Could you check a few things on this model? Use its own coordinates, in mm. Give positions to 0.01 mm unless a question says otherwise; leave off trailing zeros. Loops run counter-clockwise (first coordinate to the right, second up) from the corner with the lowest first, then second, coordinate; pieces in that order, holes last. Notation, with made-up numbers: M 19,5.25 L 58,5.25 A23 ccw 58,37.25 Z; hole C 7,28 d4. An arc over 180 degrees is marked long. Answer in a Markdown table with one row per item. Add a question column.
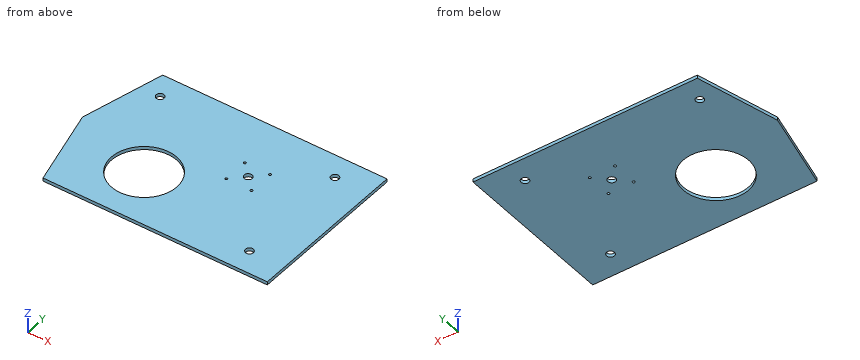
```python
from build123d import *

# Parameters (mm, degrees)
SKETCH1_R           = 40
SKETCH1_R_2         = 4.8
SKETCH1_R_3         = 1.5
BOSS_EXTRUDE3_DEPTH = 4


with BuildPart() as part:
    # Sketch1 → Boss-Extrude3 (new body)
    with BuildSketch(Plane.XY):
        Polygon((-125, -100), (150, -100), (150, 100), (-125, 100), (-150, 0), align=None)
        with Locations((-50, -33.333333333)):
            Circle(SKETCH1_R, mode=Mode.SUBTRACT)
        with Locations((107.142857143, -71.428571429)):
            Circle(SKETCH1_R_2, mode=Mode.SUBTRACT)
        with Locations((-107.142857143, 71.428571429)):
            Circle(SKETCH1_R_2, mode=Mode.SUBTRACT)
        with Locations((21.832408692, 6.152026506)):
            Circle(SKETCH1_R_3, mode=Mode.SUBTRACT)
        with Locations((37.332408692, 21.652026506)):
            Circle(SKETCH1_R_2, mode=Mode.SUBTRACT)
        with Locations((52.832408692, 6.152026506)):
            Circle(SKETCH1_R_3, mode=Mode.SUBTRACT)
        with Locations((21.832408692, 37.152026506)):
            Circle(SKETCH1_R_3, mode=Mode.SUBTRACT)
        with Locations((52.832408692, 37.152026506)):
            Circle(SKETCH1_R_3, mode=Mode.SUBTRACT)
        with Locations((107.142857143, 71.428571429)):
            Circle(SKETCH1_R_2, mode=Mode.SUBTRACT)
    extrude(amount=BOSS_EXTRUDE3_DEPTH)


solid = part.part
```
Item 1: Suppose I cut it at A-A (x = -50). List the corners of the cut face in (y, z) for me.
Item 2: For P1, Ø2.5, axis at x = 21.83, y = 6.15, coming from the +Z side, with a flat end and sliding along its axis, tell me the tip position at first contact or that it passes through.
Item 3: Suppose I cut it at C-C (z = 3.1). Give the number of separate pieces and of enclosed holes in the cut face, then the cut area to 3 significant figures.
Item 4: Suppose I cut it at D-D (y = 87). List the corners of the cut face in (x, z) for me.
Item 5: Suppose I cut it at B-B (y = -29). List the corners of the cut face in (x, z) for me, then the cut area to 3 significant figures.
Item 6: I need wall thicknesses on L1, parallel to X at y = 70, z = 3.65; L2, parallel to X at y = 67, z = 0.5; L3, parallel to Y at x = 103, z = 1.2. Which ranges of each line are inside material? Lowest first, please.
Values found:
| question | item | result |
|---|---|---|
| 1 | outline | M -100,0 L -73.33,0 L -73.33,4 L -100,4 Z; M 6.67,0 L 100,0 L 100,4 L 6.67,4 Z |
| 2 | P1 | through |
| 3 | separate pieces | 1 |
| 3 | enclosed holes | 9 |
| 3 | area | 52,200 mm² |
| 4 | outline | M -128.25,0 L 150,0 L 150,4 L -128.25,4 Z |
| 5 | outline | M -142.75,0 L -89.76,0 L -89.76,4 L -142.75,4 Z; M -10.24,0 L 150,0 L 150,4 L -10.24,4 Z |
| 5 | area | 853 mm² |
| 6 | L1 | -132.5 to -111.73, -102.56 to 102.56, 111.73 to 150 |
| 6 | L2 | -133.25 to -108.99, -105.29 to 105.29, 108.99 to 150 |
| 6 | L3 | -100 to -73.85, -69 to 69, 73.85 to 100 |
